from build123d import *

# Parameters (mm, degrees)
SKETCH_1_W          = 150
SKETCH_1_H          = 35
EXTRUDE_1_DEPTH     = 30
SKETCH_2_R          = 6
CUT_EXTRUDE_3_DEPTH = 20
SKETCH_3_W          = 80
SKETCH_3_H          = 25
CUT_EXTRUDE_2_DEPTH = 15
SKETCH_5_R          = 10
CUT_EXTRUDE_6_DEPTH = 95
SKETCH_6_R          = 6
CUT_EXTRUDE_7_DEPTH = 25


with BuildPart() as part:
    # Эскиз1 → Бобышка-Вытянуть1 (new body)
    with BuildSketch(Plane(origin=(0, 0, 0), x_dir=(1, 0, 0), z_dir=(0, 1, 0))):
        with Locations((24.604604994, 5.307565724)):
            Rectangle(SKETCH_1_W, SKETCH_1_H)
    extrude(amount=EXTRUDE_1_DEPTH)

    # Эскиз2 → Вырез-Вытянуть3 (cut)
    with BuildSketch(Plane(origin=(99.604604994, 0, 0), x_dir=(0, 0, -1), z_dir=(1, 0, 0))):
        with Locations((11.307565724, 15)):
            Circle(SKETCH_2_R)
    extrude(amount=-CUT_EXTRUDE_3_DEPTH, mode=Mode.SUBTRACT)

    # Эскиз3 → Вырез-Вытянуть2 (cut)
    with BuildSketch(Plane(origin=(0, 0, -22.807565724), x_dir=(-1, 0, 0), z_dir=(0, 0, -1))):
        with Locations((-24.604604994, 12.5)):
            Rectangle(SKETCH_3_W, SKETCH_3_H)
    extrude(amount=-CUT_EXTRUDE_2_DEPTH, mode=Mode.SUBTRACT)

    # Эскиз5 → Вырез-Вытянуть6 (cut)
    with BuildSketch(Plane(origin=(79.604604994, 0, 0), x_dir=(0, 0, -1), z_dir=(1, 0, 0))):
        with Locations((11.307565724, 15)):
            Circle(SKETCH_5_R)
    extrude(amount=-CUT_EXTRUDE_6_DEPTH, mode=Mode.SUBTRACT)

    # Эскиз6 → Вырез-Вытянуть7 (cut)
    with BuildSketch(Plane(origin=(-15.395395006, 0, 0), x_dir=(0, 0, -1), z_dir=(1, 0, 0))):
        with Locations((11.307565724, 15)):
            Circle(SKETCH_6_R)
    extrude(amount=-CUT_EXTRUDE_7_DEPTH, mode=Mode.SUBTRACT)


solid = part.part
Work out the finished part from the listing and answer in its coordinate system (mm). A direction names the side the tool comes from. Give positions to 0.01 mm unless a question says otherwise; leave off trailing zeros. Loops run counter-clockwise (first coordinate to the right, second up) from the corner with the lowest first, then second, coordinate; pieces in that order, holes last. Notation, with made-up numbers: (-14.75, 83.5) - (-9.75, 83.5) arc R19 cw to (-9.75, 89.5) - close; hole circle Ø4 at (67, -36). An arc over 180 degrees is marked (long way). Answer in a Markdown table with one row per item. Add a question column.
Q1. A tool of negligible diameter and unlimited length cuts with its end or side. For faces 5 (the cylindrical face through (-27.72, 15.264, -5.313)), 6 (the cylindrical face through (43.325, 15.44, -1.317)), 7 (the flat face through (25, 25, -15)), from which of +Z, -Z, +X, -X, +Y, -Y can it reach the whole face along a straight path? Write none if from no direction.
Q2. Determine the mould class of faces 1 (the flat face through (-40.395, 15, -11)), 2 (the cylindrical face through (89.745, 15.264, -5.313)), 3 (the flat face through (99.605, 15, -5)), 4 (the flat face through (24, 30, -6)) for opening direction Y: released by +Y, released by -Y, zero draft, split by the parting line, or undercut.
Q3. The part is cut by section B-B (x = -28.5). Determine the outline of the cut face in (y, z).
Q4. The part is cut by section A-A (y = 15). Determine the outline of the cut face in (x, z), and give its area (3 significant figures).
Q5. The part is cut by section D-D (x = 12). Determine the outline of the cut face in (y, z).
Q6. The part is cut by section C-C (z = -4). Determine the outline of the cut face in (x, y).
Q7. Each of these flat-tipped pins is pushed along its axis until it touches: P1, Ø2, axis at x = 55, z = -11, coming from the -Y side; P2, Ø4.5, axis at x = 19, y = 2.5, coming from the -Z side; P3, Ø11, axis at y = 15, z = -11.31, coming from the +X side. Where does it stop, or does it pass through?
Q8. Consider line 1 along X through (y, z) = (19.25, -18); line 2 along Y through (x, z) = (-32.5, -11); line 3 along X through (y, z) = (3, -16). Determine where each line is inside the solid, lowest interval first.
Solution:
| question | item | result |
|---|---|---|
| 1 | face 5 | +X |
| 1 | face 6 | none |
| 1 | face 7 | -Z, -Y |
| 2 | face 1 | undercut |
| 2 | face 2 | undercut |
| 2 | face 3 | zero draft |
| 2 | face 4 | released by +Y |
| 3 | outline | (0, -22.81) - (30, -22.81) - (30, 12.19) - (0, 12.19) - close; hole circle Ø12 at (15, -11.31) |
| 4 | outline | (-50.4, -22.81) - (-15.4, -22.81) - (-15.4, -17.31) - (-40.4, -17.31) - (-40.4, -5.31) - (-15.4, -5.31) - (-15.4, -1.31) - (79.6, -1.31) - (79.6, -5.31) - (99.6, -5.31) - (99.6, 12.19) - (-50.4, 12.19) - close; (64.6, -22.81) - (99.6, -22.81) - (99.6, -17.31) - (79.6, -17.31) - (79.6, -21.31) - (64.6, -21.31) - close |
| 4 | area | 2,690 mm² |
| 5 | outline | (0, -7.81) - (5.63, -7.81) arc R10 cw to (24.37, -7.81) - (25, -7.81) - (25, -22.81) - (30, -22.81) - (30, 12.19) - (0, 12.19) - close |
| 6 | outline | (-50.4, 0) - (99.6, 0) - (99.6, 30) - (-50.4, 30) - close; hole (-15.4, 8.17) - (79.6, 8.17) - (79.6, 21.83) - (-15.4, 21.83) - close |
| 7 | P1 | stops at y = 25 |
| 7 | P2 | stops at z = -7.81 |
| 7 | P3 | stops at x = -40.4 |
| 8 | line 1 | x = -50.4 to -15.4, 79.6 to 99.6 |
| 8 | line 2 | y = 0 to 9.01, 20.99 to 30 |
| 8 | line 3 | x = -50.4 to -15.4, 64.6 to 99.6 |
